```python
from build123d import *

# Parameters (mm, degrees)
SKETCH1_W           = 90.58
SKETCH1_H           = 70.48
SKETCH1_R           = 1.25
BOSS_EXTRUDE1_DEPTH = 10
SKETCH2_W           = 10
SKETCH2_H           = 4
BOSS_EXTRUDE2_DEPTH = 10
SKETCH3_W           = 10
SKETCH3_H           = 4
BOSS_EXTRUDE3_DEPTH = 10
FILLET2_R           = 2
FILLET3_R           = 2
CUT_EXTRUDE1_REACH  = 123.317
SKETCH4_R           = 1.5


with BuildPart() as part:
    # Sketch1 → Boss-Extrude1 (new body)
    with BuildSketch(Plane(origin=(0, 0, 0), x_dir=(1, 0, 0), z_dir=(0, 1, 0))):
        with Locations((-45.29, -35.24)):
            Rectangle(SKETCH1_W, SKETCH1_H)
        with Locations(Location((-3.505, -67.355, 0), (0, 0, 270))):
            Circle(SKETCH1_R, mode=Mode.SUBTRACT)
        with BuildLine():
            Line((-83.7, -61.178989341), (-83.7, -3.9))
            Line((-83.7, -3.9), (-6.990565569, -3.9))
            ThreePointArc((-6.990565569, -3.9), (-6.996312077, -5.25078698), (-6.49, -6.503107452))
            Line((-6.49, -6.503107452), (-6.49, -64.91))
            Line((-6.49, -64.91), (-81.134920114, -64.91))
            ThreePointArc((-81.134920114, -64.91), (-81.937140101, -62.714273406), (-83.7, -61.178989341))
        make_face(mode=Mode.SUBTRACT)
        with Locations(Location((-87.32, -4.06, 0), (0, 0, 270))):
            Circle(SKETCH1_R, mode=Mode.SUBTRACT)
        with Locations(Location((-3.56, -4.59, 0), (0, 0, 270))):
            Circle(SKETCH1_R, mode=Mode.SUBTRACT)
        with Locations(Location((-85.8, -65.37, 0), (0, 0, 270))):
            Circle(SKETCH1_R, mode=Mode.SUBTRACT)
    extrude(amount=-BOSS_EXTRUDE1_DEPTH)

    # Sketch2 → Boss-Extrude2 (add)
    with BuildSketch(Plane.XY.offset(70.48)):
        with Locations((-85.58, -8)):
            Rectangle(SKETCH2_W, SKETCH2_H)
        with Locations((-5, -8)):
            Rectangle(SKETCH2_W, SKETCH2_H)
    extrude(amount=BOSS_EXTRUDE2_DEPTH)

    # Sketch3 → Boss-Extrude3 (add)
    with BuildSketch(Plane(origin=(0, 0, 0), x_dir=(-1, 0, 0), z_dir=(0, 0, -1))):
        with Locations((5, -8)):
            Rectangle(SKETCH3_W, SKETCH3_H)
        with Locations((85.58, -8)):
            Rectangle(SKETCH3_W, SKETCH3_H)
    extrude(amount=BOSS_EXTRUDE3_DEPTH)

    # Fillet2
    fillet2_edges = [part.edges().sort_by_distance(p)[0] for p in [
        (-90.58, -8, 80.48),
        (-80.58, -8, 80.48),
        (0, -8, 80.48),
        (-10, -8, 80.48),
        (0, -8, -10),
        (-10, -8, -10),
        (-90.58, -8, -10),
        (-80.58, -8, -10),
    ]]
    fillet(fillet2_edges, radius=FILLET2_R)

    # Fillet3
    fillet3_edges = [part.edges().sort_by_distance(p)[0] for p in [
        (-85.58, -6, 80.48),
        (-90.58, -6, 74.48),
        (-80.58, -6, 74.48),
        (-89.994213562, -6, 79.894213562),
        (-81.165786438, -6, 79.894213562),
        (-90.58, -6, -4),
        (-85.58, -6, -10),
        (-80.58, -6, -4),
        (-81.165786438, -6, -9.414213562),
        (-89.994213562, -6, -9.414213562),
        (-5, -6, -10),
        (-10, -6, -4),
        (-9.414213562, -6, -9.414213562),
        (-0.585786438, -6, -9.414213562),
        (-5, -6, 80.48),
        (-10, -6, 74.48),
        (0, -6, 74.48),
        (-9.414213562, -6, 79.894213562),
        (-0.585786438, -6, 79.894213562),
        (0, -6, -4),
    ]]
    fillet(fillet3_edges, radius=FILLET3_R)

    # Sketch4 → Cut-Extrude1 (cut, up to next)
    with BuildSketch(Plane(origin=(0, -6, 0), x_dir=(1, 0, 0), z_dir=(0, 1, 0)), mode=Mode.PRIVATE) as cut_extrude1_sk1:
        with Locations(Location((-5, 4, 0), (0, 0, 270))):
            Circle(SKETCH4_R)
    cut_extrude1_tool1 = extrude(cut_extrude1_sk1.sketch, amount=-CUT_EXTRUDE1_REACH, mode=Mode.PRIVATE) & part.part
    # Sketch4 → Cut-Extrude1 (cut, up to next)
    with BuildSketch(Plane(origin=(0, -6, 0), x_dir=(1, 0, 0), z_dir=(0, 1, 0)), mode=Mode.PRIVATE) as cut_extrude1_sk2:
        with Locations(Location((-5, -74.48, 0), (0, 0, 270))):
            Circle(SKETCH4_R)
    cut_extrude1_tool2 = extrude(cut_extrude1_sk2.sketch, amount=-CUT_EXTRUDE1_REACH, mode=Mode.PRIVATE) & part.part
    # Sketch4 → Cut-Extrude1 (cut, up to next)
    with BuildSketch(Plane(origin=(0, -6, 0), x_dir=(1, 0, 0), z_dir=(0, 1, 0)), mode=Mode.PRIVATE) as cut_extrude1_sk3:
        with Locations(Location((-85.58, -74.48, 0), (0, 0, 270))):
            Circle(SKETCH4_R)
    cut_extrude1_tool3 = extrude(cut_extrude1_sk3.sketch, amount=-CUT_EXTRUDE1_REACH, mode=Mode.PRIVATE) & part.part
    # Sketch4 → Cut-Extrude1 (cut, up to next)
    with BuildSketch(Plane(origin=(0, -6, 0), x_dir=(1, 0, 0), z_dir=(0, 1, 0)), mode=Mode.PRIVATE) as cut_extrude1_sk4:
        with Locations(Location((-85.58, 4, 0), (0, 0, 270))):
            Circle(SKETCH4_R)
    cut_extrude1_tool4 = extrude(cut_extrude1_sk4.sketch, amount=-CUT_EXTRUDE1_REACH, mode=Mode.PRIVATE) & part.part
    add(cut_extrude1_tool1.solids().sort_by_distance((-5, -6, -4))[0], mode=Mode.SUBTRACT)
    add(cut_extrude1_tool2.solids().sort_by_distance((-5, -6, 74.48))[0], mode=Mode.SUBTRACT)
    add(cut_extrude1_tool3.solids().sort_by_distance((-85.58, -6, 74.48))[0], mode=Mode.SUBTRACT)
    add(cut_extrude1_tool4.solids().sort_by_distance((-85.58, -6, -4))[0], mode=Mode.SUBTRACT)


solid = part.part
```
Here's how the part is built. I have some questions about the finished solid (model axes, mm). A direction names the side the tool comes from. Give positions to 0.01 mm unless a question says otherwise; leave off trailing zeros. Order: outer loops, then holes, each group sorted by start corner. A loop starts at its lowest first (then second) coordinate and runs counter-clockwise, first axis right, second up. Notation, with made-up numbers: M 18,-1.5 L 40,-1.5 A18 cw 40,28.5 Z; hole C -7.5,85.25 d2. An arc over 180 degrees is marked long. Use a Markdown table: item, result. Add a question column.
1. Suppose I cut it at D-D (y = -4.75). List the corners of the cut face in (x, z) for me (3 decimals).
2. For pin 1 Ø5 at (x, y) = (-43.5, -4.5) entering from -Z; pin 2 Ø6.5 at (x, z) = (-6, 74) entering from +Y, each with a flat end and sliding along its axis, tell me the tip position at first contact or that it passes through.
3. I need wall thicknesses on probe 1 along X at (y, z) = (-8.65, -4); probe 2 along X at (y, z) = (-4, 21.5); probe 3 along Z at (x, y) = (-44, -4.5). Which ranges of each line are inside material? Lowest first, please. Write a range as from..to.
4. On a 3-axis mill with a long thin cutter (end or side, diameter ignored), from which of +Z, -Z, +X, -X, +Y, -Y can I reach the whole of each face in a straight line? I mean faces 5 (the flat face through (-90.58, -5, 35)), 6 (the flat face through (-6.49, -5, 35)), 7 (the flat face through (-87, -6, 73.5)), 8 (the cylindrical face through (-81.18, -8.99, -9.43)), 9 (the cylindrical face through (-9.4, -6.57, -3.94)). Say none if no direction works.
5. If we mould it in two halves opening along X, with no side actions, what happens to faces 1 (the cylindrical face through (-90.01, -8.99, -9.4)), 2 (the flat face through (-46, -5, 70.48)), 3 (the cylindrical face through (-0.6, -6.57, 74.42)), 4 (the cylindrical face through (-4.039, -4.93, 5.745))? For each: +X half, -X half, draft (parallel to the pull), parting line (faces both ways), or undercut.
6. Suppose I cut it at A-A (x = -62). List the corners of the cut face in (y, z) for me, and give its area (3 significant figures).
7. Suppose I cut it at B-B (z = 14). List the corners of the cut face in (x, y) for me.
8. Suppose I cut it at C-C (z = 74.48). List the corners of the cut face in (x, y) for me.
Results list:
| question | item | result |
|---|---|---|
| 1 | outline | M -90.58,0 L 0,0 L 0,70.48 L -90.58,70.48 Z; hole C -87.32,4.06 d2.5; hole C -85.8,65.37 d2.5; hole M -83.7,3.9 L -6.991,3.9 A3.499 cw -6.49,6.503 L -6.49,64.91 L -81.135,64.91 A4.688 cw -83.7,61.179 Z; hole C -3.56,4.59 d2.5; hole C -3.505,67.355 d2.5 |
| 2 | pin 1 | stops at z = 0 |
| 2 | pin 2 | stops at y = -6 |
| 3 | probe 1 | x = -90.58..-87.08, -84.08..-80.58, -10..-6.5, -3.5..0 |
| 3 | probe 2 | x = -90.58..-83.7, -6.49..0 |
| 3 | probe 3 | z = 0..3.9, 64.91..70.48 |
| 4 | face 5 | +Z, -Z, -X, +Y, -Y |
| 4 | face 6 | +Y, -Y |
| 4 | face 7 | +Z, +X, -X, +Y |
| 4 | face 8 | -Z, +Y, -Y |
| 4 | face 9 | -Z, +Y |
| 5 | face 1 | -X half |
| 5 | face 2 | undercut |
| 5 | face 3 | +X half |
| 5 | face 4 | undercut |
| 6 | outline | M -10,0 L 0,0 L 0,3.9 L -10,3.9 Z; M -10,64.91 L 0,64.91 L 0,70.48 L -10,70.48 Z |
| 6 | area | 94.7 mm² |
| 7 | outline | M -90.58,-10 L -83.7,-10 L -83.7,0 L -90.58,0 Z; M -6.49,-10 L 0,-10 L 0,0 L -6.49,0 Z |
| 8 | outline | M -90.58,-10 L -87.08,-10 L -87.08,-6 L -88.58,-6 A2 ccw -90.58,-8 Z; M -84.08,-10 L -80.58,-10 L -80.58,-8 A2 ccw -82.58,-6 L -84.08,-6 Z; M -10,-10 L -6.5,-10 L -6.5,-6 L -8,-6 A2 ccw -10,-8 Z; M -3.5,-10 L 0,-10 L 0,-8 A2 ccw -2,-6 L -3.5,-6 Z |
